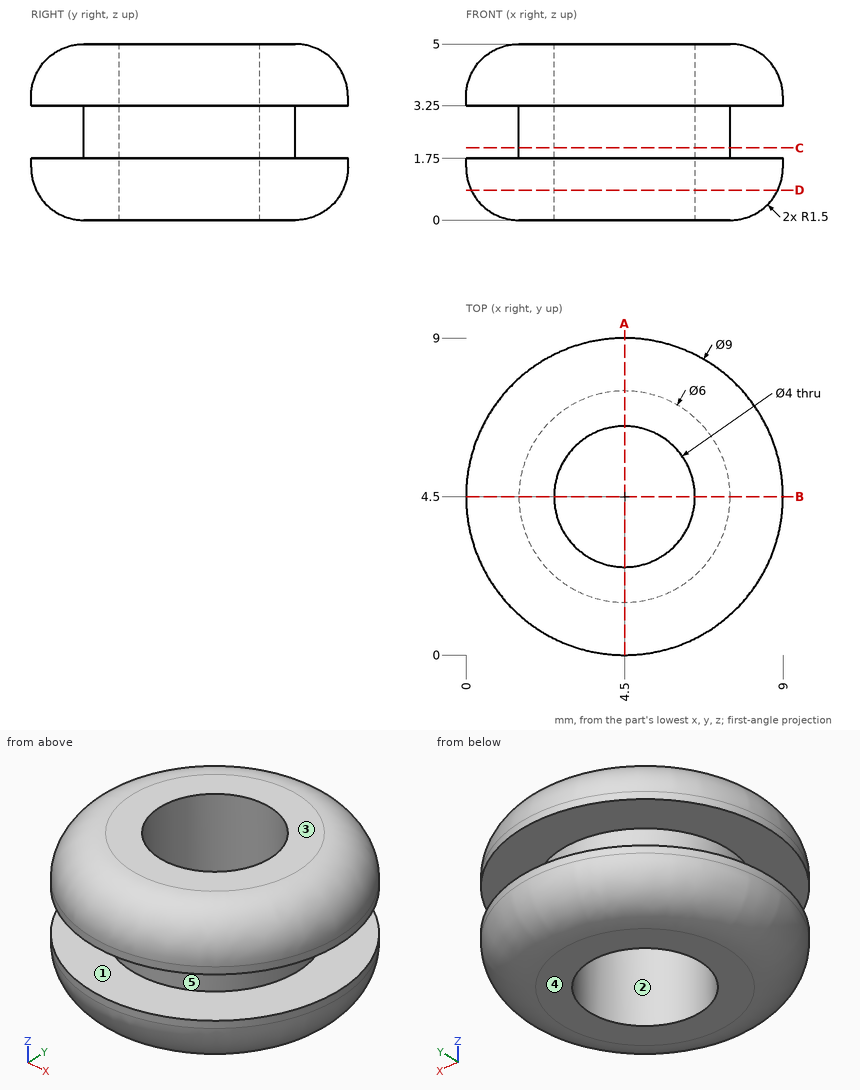
Geometry check sheet. Reference: drawing and pictorial views, mm from the part's lowest x, y, z. A direction names the side the tool comes from. Coordinates: 2 decimals unless noted, no trailing zeros. Write each loop counter-clockwise with the first axis right and the second up, starting at its lowest first coordinate (ties: lowest second). Pieces come first, ordered by that corner, then holes. Notation, with made-up numbers: M 54,4 L 64,4 A14 ccw 64,11 Z; hole C 75,27.25 d10. An arc over 180 degrees is marked long. One line per question, with ' | ' between items.
1) Material ranges on L1, parallel to Y at x = 4.5, z = 3.55; L2, parallel to Y at x = 4.5, z = 3.15; L3, parallel to Z at x = 1.5, y = 5, recorded low to high.
Solutions:
L1: 0 to 2.5, 6.5 to 9 | L2: 1.5 to 2.5, 6.5 to 7.5 | L3: 0 to 1.75, 3.25 to 5
2) Access from +Z, -Z, +X, -X, +Y, -Y to the whole of each face (thin tool, end or side, straight path). Record for the marked faces 1 and 2.
Solutions:
face 1: none | face 2: +Z, -Z
3) Depth check by flat-ended pin: pin 1 Ø1.5 at (x, y) = (4.5, 4) entering from -Z (3 decimals); pin 2 Ø2 at (y, z) = (6, 3) entering from -X. Enter the tip coordinate at first touch or a pass-through.
Solutions:
pin 1: through | pin 2: x = 0.03
4) Sectioned sample at D-D on z = 0.85. Record the cut outline in (x, y), then the cut area to 3 significant figures.
Solutions:
outline: C 4.5,4.5 d8.7; hole C 4.5,4.5 d4 | area: 46.9 mm^2
5) Sectioned sample at A-A on x = 4.5. Record the cut outline in (y, z), then the cut area to 3 significant figures.
Solutions:
outline: M 0,1.5 A1.5 ccw 1.5,0 L 2.5,0 L 2.5,5 L 1.5,5 A1.5 ccw 0,3.5 L 0,3.25 L 1.5,3.25 L 1.5,1.75 L 0,1.75 Z; M 6.5,0 L 7.5,0 A1.5 ccw 9,1.5 L 9,1.75 L 7.5,1.75 L 7.5,3.25 L 9,3.25 L 9,3.5 A1.5 ccw 7.5,5 L 6.5,5 Z | area: 18.6 mm^2
6) Sectioned sample at C-C on z = 2.05. Record the cut outline in (x, y), then the cut area to 3 significant figures.
Solutions:
outline: C 4.5,4.5 d6; hole C 4.5,4.5 d4 | area: 15.7 mm^2
7) Release check for a two-part mould opening along Z. For the marked faces 3, 4 and 5 record: +Z half, -Z half, draft (parallel to the pull), parting line (faces both ways), or undercut.
Solutions:
face 3: +Z half | face 4: -Z half | face 5: undercut
